from build123d import *

# Parameters (mm, degrees)
F1_DEPTH = 63.5
F0_W     = 25.4
F0_H     = 19.05
F2_DEPTH = 12.7
F3_DEPTH = 7.9375
F5_R     = 6.35
F6_R     = 6.35
F7_R     = 6.35


with BuildPart() as f1:
    # F0 (on Front) → F1 (new body, symmetric)
    with BuildSketch(Plane.XZ):
        Polygon((40.64, -9.525), (40.64, 9.525), (21.59, 9.525), (-40.64, 9.525), (-40.64, -9.525), align=None)
    extrude(amount=F1_DEPTH, both=True)

    # F0 (on Front) → F2 (join, symmetric)
    with BuildSketch(Plane.XZ):
        with BuildLine():
            Line((21.59, 9.525), (40.64, 9.525))
            Line((40.64, 9.525), (40.64, 27.0002))
            ThreePointArc((40.64, 27.0002), (45.2896798487, 38.2255201513), (56.515, 42.8752))
            Line((56.515, 42.8752), (59.69, 42.8752))
            Line((59.69, 42.8752), (59.69, 61.9252))
            Line((59.69, 61.9252), (56.515, 61.9252))
            add(Edge.make_bspline(
                [(54.6273008741, 61.8741475398), (55.2538493606, 61.8930466239), (55.8830864872, 61.910065703), (56.515, 61.9252)],
                knots=[109.2371612745, 109.2371612745, 109.2371612745, 109.2371612745, 110.3851212122, 110.3851212122, 110.3851212122, 110.3851212122], degree=3))
            ThreePointArc((54.6273008741, 61.8741475398), (31.1606757438, 51.01923134), (21.59, 27.0002))
            Line((21.59, 27.0002), (21.59, 9.525))
        make_face()
        with Locations((72.39, 52.4002)):
            Rectangle(F0_W, F0_H)
    extrude(amount=F2_DEPTH, both=True)

    # F0 (on Front) → F3 (join, symmetric)
    with BuildSketch(Plane.XZ):
        with BuildLine():
            Line((-40.64, 9.525), (21.59, 9.525))
            Line((21.59, 9.525), (21.59, 27.0002))
            ThreePointArc((21.59, 27.0002), (31.1606757438, 51.01923134), (54.6273008741, 61.8741475398))
            add(Edge.make_bspline(
                [(-40.64, 9.525), (-40.2688790692, 41.2539616871), (-4.9935759741, 60.0757552579), (54.6273008741, 61.8741475398)],
                knots=[0, 0, 0, 0, 109.2371612745, 109.2371612745, 109.2371612745, 109.2371612745], degree=3))
        make_face()
    extrude(amount=F3_DEPTH, both=True)

    # F0 (on Front) → F4 (revolve)
    with BuildSketch(Plane.XZ):
        Polygon((85.09, 61.9252), (85.09, 42.8752), (85.09, 38.1), (110.49, 38.1), (110.49, 66.675), (85.09, 66.675), align=None)
    revolve(axis=Axis((85.09, 0, 52.3875), (0, 0, 1)))

    # F5
    f5_edges = [f1.edges().sort_by_distance(p)[0] for p in [
        (40.64, -63.5, 0),
    ]]
    fillet(f5_edges, radius=F5_R)

    # F6
    f6_edges = [f1.edges().sort_by_distance(p)[0] for p in [
        (-40.64, -63.5, 0),
    ]]
    fillet(f6_edges, radius=F6_R)

    # F7
    f7_edges = [f1.edges().sort_by_distance(p)[0] for p in [
        (40.64, 63.5, 0),
        (-40.64, 63.5, 0),
    ]]
    fillet(f7_edges, radius=F7_R)


solid = f1.part
Can you work these out from the model? Positions are in its coordinate system, mm. A direction names the side the tool comes from. Give positions to 0.01 mm unless a question says otherwise; leave off trailing zeros. Loops run counter-clockwise (first coordinate to the right, second up) from the corner with the lowest first, then second, coordinate; pieces in that order, holes last. Notation, with made-up numbers: (86.25, 32) - (103.25, 32) arc R21 ccw to (103.25, 62) - close; hole circle Ø5 at (49, 59). An arc over 180 degrees is marked (long way). Answer as a JSON object with one key per item and string values.
Q1. If we mould it in two halves opening along X, with no side actions, what happens to faces 1 (the flat face through (21.59, 10, 18)), 2 (the cylindrical face through (45.167, -0.178, 38.101)), 3 (the flat face through (85, 0, 38.1))? For each: pulls with the +X half, pulls with the -X half, needs draft (parallel to the pull), parting line crosses it, or undercut.
Geometry says:
{"face 1": "pulls with the -X half", "face 2": "undercut", "face 3": "needs draft"}
Q2. If I drill on L1, parallel to Y at x = 4.5, z = 20; L2, parallel to Y at x = 35.5, z = 43.5; L3, parallel to Z at x = 86, y = -4 (3 decimals), over which ranges is the centre line in solid material (lowest first)?
Geometry says:
{"L1": "-7.94 to 7.94", "L2": "-12.7 to 12.7", "L3": "38.1 to 66.675"}
Q3. Imagine slicing it at B-B on y = -21. Write out the boundary of the cut face in (x, z) (3 decimals).
Geometry says:
{"outline": "(-40.64, -9.525) - (40.64, -9.525) - (40.64, 9.525) - (-40.64, 9.525) - close; (70.802, 38.1) - (99.378, 38.1) - (99.378, 66.675) - (70.802, 66.675) - close"}
Q4. Imagine slicing it at D-D on x = 85.09. Write out the boundary of the cut face in (y, z) (3 decimals), plus the area to 3 significant figures.
Geometry says:
{"outline": "(-25.4, 38.1) - (25.4, 38.1) - (25.4, 66.675) - (-25.4, 66.675) - close", "area": "1,450 mm²"}
Q5. Will these pins go through, and if not, where does the flat tip stop? P1, Ø12.5, axis at x = 39.5, z = 42.5, coming from the -Y side; P2, Ø12, axis at x = 44, y = -20, coming from the +Z side (3 decimals); P3, Ø4, axis at y = -11, z = 19, coming from the -X side.
Geometry says:
{"P1": "y = -12.7", "P2": "z = 9.525", "P3": "x = 21.59"}
Q6. Which directions (+Z, -Z, +X, -X, +Y, -Y) give clear straight access to the entire face, cutting with the end or side of a thin tool? Please do faces 4 (the flat face through (-4, -7.938, 30)), 5 (the flat face through (40.64, -1, 4)), 6 (the flat face through (59, 0, 42.875)), 7 (the flat face through (37, 12.7, 36)).
Geometry says:
{"face 4": "+Z, -X, -Y", "face 5": "-Z, +X, +Y, -Y", "face 6": "-Z", "face 7": "+Z, -X, +Y"}
Q7. Imagine slicing it at C-C on y = -50. Write out the boundary of the cut face in (x, z) (3 decimals), plus the area to 3 significant figures.
Geometry says:
{"outline": "(-40.64, -9.525) - (40.64, -9.525) - (40.64, 9.525) - (-40.64, 9.525) - close", "area": "1,550 mm²"}
Q8. Imagine slicing it at A-A on z = 3.5. Write out the boundary of the cut face in (x, y).
Geometry says:
{"outline": "(-40.64, -57.15) arc R6.35 ccw to (-34.29, -63.5) - (34.29, -63.5) arc R6.35 ccw to (40.64, -57.15) - (40.64, 57.15) arc R6.35 ccw to (34.29, 63.5) - (-34.29, 63.5) arc R6.35 ccw to (-40.64, 57.15) - close"}
